Autodesk Inventor part; units mm, degrees
ref_plane "Work Plane1" through (0, 0, 11) normal (0, 0, 1) x (1, 0, 0)
ref_plane "YZ Plane" through (0, 0, 0) normal (1, 0, 0) x (0, 1, 0)
ref_plane "XZ Plane" through (0, 0, 0) normal (0, 1, 0) x (-1, 0, 0)
sketch "Sketch1" plane through (0, 0, 0) normal (1, 0, 0) x (0, 1, 0)
  circle A0 centre (0, 0) radius 11
  dimension "d0" = 22
extrude "Extrusion1" add sketch "Sketch1" along normal blind 38
sketch "Sketch2" plane through (38, 0, 0) normal (1, 0, 0) x (0, 0, -1)
  circle A0 centre (0, 0) radius 7.5
  dimension "d3" = 15
extrude "Extrusion2" add sketch "Sketch2" along normal blind 5
ref_plane "Work Plane1" through (0, 0, 11) normal (0, 0, 1) x (1, 0, 0)
sketch "Sketch3" plane through (0, 0, 11) normal (0, 0, 1) x (1, 0, 0)
  line L0 (0, 0) -> (19, 0) construction
  circle A0 centre (19, 0) radius 4.7625
  dimension "d7" = 19
  dimension "d8" = 9.525
extrude "Extrusion3" cut sketch "Sketch3" against normal blind 22
sketch "Sketch4" plane through (43, 0, 0) normal (1, 0, 0) x (0, 0, -1)
  circle A0 centre (0, 0) radius 9.525
  dimension "d11" = 19.05
extrude "Extrusion4" add sketch "Sketch4" along normal blind 157
sketch "Sketch5" plane through (200, 0, 0) normal (1, 0, 0) x (0, 0, -1)
  circle A0 centre (0, 0) radius 7.5
  dimension "d14" = 15
extrude "Extrusion5" add sketch "Sketch5" along normal blind 30
chamfer "Chamfer1" distance 7.5 angle 60 1 edges at (230, 0, 7.5) measured on face at (230, -0.5635, 2.141)
thread "Thread1"
properties part number "parafuso"
Build history of the part. All positions in model axes, mm. A direction names the side the tool comes from. Round coordinates to 2 decimals unless told otherwise and drop trailing zeros. Loops run counter-clockwise (first coordinate to the right, second up) from the corner with the lowest first, then second, coordinate; pieces in that order, holes last. Notation, with made-up numbers: (-36, 23) -> (23, 23) arc R11 ccw to (23, 35) -> close; hole circle Ø11 at (11.25, 20.25). An arc over 180 degrees is marked (long way). Use CSV: the item, a comma, the result in double quotes. Start each with the question number.
Q1. Saw through at A-A on x = 145.5. Give the cut face in (y, z) (3 decimals).
Q2. Saw through at B-B on x = 19. Give the cut face in (y, z), and give its area (3 significant figures).
Q3. Drill centre lines: L1, parallel to Y at x = 19, z = 1; L2, parallel to Y at x = 19, z = -5.5; L3, parallel to X at y = 9.75, z = -2.75. Where is each one in solid material? Low to high.
Q4. Which spindle directions (+Z, -Z, +X, -X, +Y, -Y) get a long thin tool onto all of the face, cutting with end or side? Do faces 1 (the face through (38, 7.2, 2.6)), 2 (the face through (120.401, 5.796, 7.559)), 3 (the face through (18.734, 5.076, 9.759)). Say none if no direction does.
Q5. Flat gauge pins, fed straight in: pin 1 Ø5 at (x, y) = (172, -7.5) entering from +Z; pin 2 Ø12 at (y, z) = (-3, 6) entering from +X; pin 3 Ø6.5 at (y, z) = (3.5, -0.5) entering from +X. Where does each tip first touch, or does it go through?
Q6. Mould opens along X. For faces 4 (the face through (224.86, 2.9, 0.64)), 5 (the face through (0, 0, 0)), 6 (the face through (14.242, 0.209, 0.154)) say: +X half, -X half, draft (parallel to the pull), parting line (faces both ways), or undercut.
Solutions:
1,outline,"circle Ø19.05 at (0, 0)"
2,outline,"(-4.76, -9.92) -> (-4.76, 9.92) arc R11 ccw to start; (4.76, -9.92) arc R11 ccw to (4.76, 9.92) -> close"
2,area,"177 mm^2"
3,L1,"y = -10.95 to -4.76, 4.76 to 10.95"
3,L2,"y = -9.53 to -4.76, 4.76 to 9.53"
3,L3,"x = 0 to 38"
4,face 1,"none"
4,face 2,"+X"
4,face 3,"+X, -X"
5,pin 1,"stops at z = 8.11"
5,pin 2,"stops at x = 228.77"
5,pin 3,"stops at x = 229.51"
6,face 4,"+X half"
6,face 5,"-X half"
6,face 6,"undercut"
